```python
from build123d import *

# Parameters (mm, degrees)
F0_R     = 16
F0_R_2   = 7.55
F1_DEPTH = 100
F2_R     = 5
F3_R     = 3


with BuildPart() as f1:
    # F0 (on Front) → F1 (new body)
    with BuildSketch(Plane.XZ):
        Circle(F0_R)
        Circle(F0_R_2, mode=Mode.SUBTRACT)
    extrude(amount=F1_DEPTH)

    # F2
    f2_edges = [f1.edges().sort_by_distance(p)[0] for p in [
        (-16, -100, 0),
        (-16, 0, 0),
    ]]
    fillet(f2_edges, radius=F2_R)

    # F3
    f3_edges = [f1.edges().sort_by_distance(p)[0] for p in [
        (-7.55, 0, 0),
    ]]
    fillet(f3_edges, radius=F3_R)


solid = f1.part
```
Here's how the part is built. I have some questions about the finished solid (model axes, mm). Give positions to 0.01 mm unless a question says otherwise; leave off trailing zeros. Write each loop counter-clockwise with the first axis right and the second up, starting at its lowest first coordinate (ties: lowest second). Pieces come first, ordered by that corner, then holes. Notation, with made-up numbers: (-5, -17.75) -> (40, -17.75) arc R27 ccw to (40, 7.25) -> close; hole circle Ø8 at (-28.75, -10.75). An arc over 180 degrees is marked (long way). Use one line per item in the form item = value.
1) If I drill on L1, parallel to Z at x = -0.5, y = -76; L2, parallel to X at y = -78.5, z = 5.5; L3, parallel to X at y = -68, z = 1, over which ranges is the centre line in solid material (lowest first)? Write a range as [from, to].
Verdict:
L1 = [-15.99, -7.53], [7.53, 15.99]
L2 = [-15.02, -5.17], [5.17, 15.02]
L3 = [-15.97, -7.48], [7.48, 15.97]
2) Suppose I cut it at C-C (y = -73). Please give me the cut outline in (x, z), and give its area (3 significant figures).
Verdict:
outline = circle Ø32 at (0, 0); hole circle Ø15.1 at (0, 0)
area = 625 mm2
3) Suppose I cut it at B-B (x = 0). Please give me the cut outline in (y, z).
Verdict:
outline = (-100, -11) arc R5 ccw to (-95, -16) -> (-5, -16) arc R5 ccw to (0, -11) -> (0, -10.55) arc R3 ccw to (-3, -7.55) -> (-100, -7.55) -> close; (-100, 7.55) -> (-3, 7.55) arc R3 ccw to (0, 10.55) -> (0, 11) arc R5 ccw to (-5, 16) -> (-95, 16) arc R5 ccw to (-100, 11) -> close
4) I'm going to push flat-ended pins straight in: pin 1 (2 mm diameter, centred on y = -34.5, z = 7, fed in from +X); pin 2 (6 mm diameter, centred on y = -31.5, z = 12, fed in from -X); pin 3 (1.5 mm diameter, centred on x = -3, z = -7.5, fed in from +Y). Where does each tip first touch, or does it pass through?
Verdict:
pin_1 = 14.83
pin_2 = -13.23
pin_3 = -0.54
5) We'd pull the mould along X, two halves only. Please class faces 1 (the face through (-1.64, -50.82, -7.37)), 2 (the face through (9, 0, -6)), 3 (the face through (-3.47, -49.37, -15.62)): +X half, -X half, draft (parallel to the pull), parting line (faces both ways), or undercut.
Verdict:
face_1 = undercut
face_2 = draft
face_3 = parting line
6) Suppose I cut it at A-A (z = 0). Please give me the cut outline in (x, y).
Verdict:
outline = (-16, -95) arc R5 ccw to (-11, -100) -> (-7.55, -100) -> (-7.55, -3) arc R3 ccw to (-10.55, 0) -> (-11, 0) arc R5 ccw to (-16, -5) -> close; (7.55, -100) -> (11, -100) arc R5 ccw to (16, -95) -> (16, -5) arc R5 ccw to (11, 0) -> (10.55, 0) arc R3 ccw to (7.55, -3) -> close
